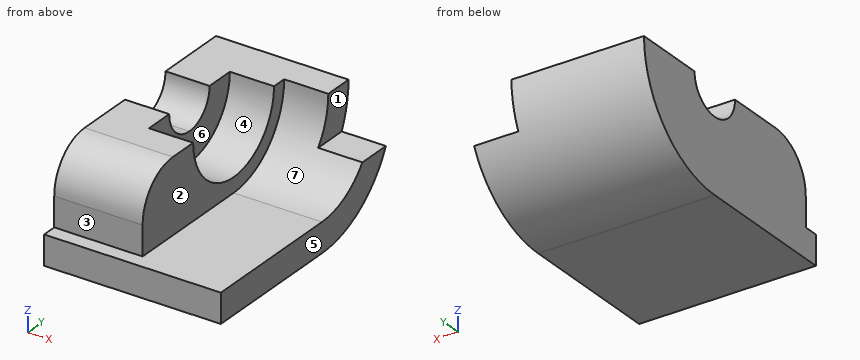
from build123d import *

# Parameters (mm, degrees)
SKETCH1_W           = 2
SKETCH1_H           = 1
BOSS_EXTRUDE1_DEPTH = 12
SKETCH2_W           = 3
SKETCH2_H           = 3
CUT_EXTRUDE1_DEPTH  = 22
CUT_EXTRUDE2_DEPTH  = 6
SKETCH4_R           = 4
CUT_EXTRUDE3_DEPTH  = 3


with BuildPart() as part:
    # Sketch1 → Boss-Extrude1 (new body)
    with BuildSketch(Plane(origin=(0, 0, 0), x_dir=(0, 0, -1), z_dir=(1, 0, 0))):
        with BuildLine():
            Line((1.5, -8), (3.5, -8))
            Line((3.5, -8), (3.5, 1))
            ThreePointArc((3.5, 1), (1.449747468, 5.949747468), (-3.5, 8))
            Line((-3.5, 8), (-3.5, 3))
            ThreePointArc((-3.5, 3), (-2.085786438, 2.414213562), (-1.5, 1))
            ThreePointArc((-1.5, 1), (-2.085786438, -0.414213562), (-3.5, -1))
            Line((-3.5, -1), (-3.5, -5))
            ThreePointArc((-3.5, -5), (-2.621320344, -7.121320344), (-0.5, -8))
            Line((-0.5, -8), (1.5, -8))
        make_face()
        with Locations((2.5, -8.5)):
            Rectangle(SKETCH1_W, SKETCH1_H)
    extrude(amount=BOSS_EXTRUDE1_DEPTH)

    # Sketch2 → Cut-Extrude1 (cut)
    with BuildSketch(Plane.XZ.offset(9)):
        with Locations((10.5, 2)):
            Rectangle(SKETCH2_W, SKETCH2_H)
    extrude(amount=-CUT_EXTRUDE1_DEPTH, mode=Mode.SUBTRACT)

    # Sketch3 → Cut-Extrude2 (cut)
    with BuildSketch(Plane(origin=(12, 0, 0), x_dir=(0, 0, -1), z_dir=(1, 0, 0))):
        with BuildLine():
            Line((1.5, 1), (1.5, -8.778964662))
            ThreePointArc((1.5, -8.778964662), (-3.5, -13.778964662), (-8.5, -8.778964662))
            Line((-8.5, -8.778964662), (-8.5, 1))
            ThreePointArc((-8.5, 1), (-3.5, 6), (1.5, 1))
        make_face()
    extrude(amount=-CUT_EXTRUDE2_DEPTH, mode=Mode.SUBTRACT)

    # Sketch4 → Cut-Extrude3 (cut)
    with BuildSketch(Plane(origin=(6, 0, 0), x_dir=(0, 0, -1), z_dir=(1, 0, 0))):
        with Locations((-3.5, 1)):
            Circle(SKETCH4_R)
    extrude(amount=-CUT_EXTRUDE3_DEPTH, mode=Mode.SUBTRACT)


solid = part.part
Design review of the part built by this model. Coordinates are the model's own, in mm. Face numbers are marked on the shaded views. A direction names the side the tool comes from. Round coordinates to 2 decimals unless told otherwise and drop trailing zeros. Write each loop counter-clockwise with the first axis right and the second up, starting at its lowest first coordinate (ties: lowest second). Pieces come first, ordered by that corner, then holes.
Item 1: Wall thickness on L1, parallel to Z at x = 10.5, y = -3; L2, parallel to Y at x = 4.25, z = 2.75; L3, parallel to X at y = -4.75, z = 0.25: over which ranges is each line inside the solid? List them lowest first.
Item 2: Consider section A-A on z = 3. Give the boundary of the cut face in (x, y), and give its area (3 significant figures).
Item 3: For pin 1 Ø1 at (x, z) = (9, 2) entering from -Y; pin 2 Ø3 at (y, z) = (3, 1.5) entering from +X; pin 3 Ø1.6 at (x, z) = (2, -0.5) entering from -Y, all flat-tipped, find the tip position at first contact; note any pin that passes through.
Item 4: Consider section D-D on x = 6.5. Give the boundary of the cut face in (y, z).
Item 5: Draft analysis for pull direction Y (two halves, no side actions). For the marked faces 5, 6 and 7, state which applies: released by +Y, released by -Y, zero draft, split by the parting line, or undercut.
Item 6: For the marked faces 1, 2, 3 and 4, list the 3-axis set-ups (+Z, -Z, +X, -X, +Y, -Y) from which the entire face can be reached by the end or side of a thin tool; tool diameter is ignored.
Item 7: Consider section C-C on y = -4. Give the boundary of the cut face in (x, z), and give its area (3 significant figures).
Item 8: Consider section B-B on x = 4.5. Give the boundary of the cut face in (y, z).
Check values:
1. L1: z = -3.5 to -1.5
1. L2: y = -6.98 to -2.93, 4.93 to 7.96
1. L3: x = 0 to 6
2. outline: (0, -6.66) - (6, -6.66) - (6, -2.97) - (3, -2.97) - (3, -0.94) - (0, -0.94) - close; (0, 2.94) - (3, 2.94) - (3, 4.97) - (6, 4.97) - (6, 5.97) - (9, 5.97) - (9, 7.98) - (0, 7.98) - close
2. area: 58.4 mm2
3. pin 1: stops at y = 5.58
3. pin 2: stops at x = 6
3. pin 3: stops at y = -8
4. outline: (-9, -3.5) - (1, -3.5) arc R7 ccw to (8, 3.5) - (6, 3.5) arc R5 cw to (1, -1.5) - (-9, -1.5) - close
5. face 5: zero draft
5. face 6: undercut
5. face 7: released by -Y
6. face 1: +Z, +X, +Y, -Y
6. face 2: +Z, +X, -Y
6. face 3: +Z, +X, -X, -Y
6. face 4: +Z, +X
7. outline: (0, -3.5) - (12, -3.5) - (12, -1.5) - (6, -1.5) - (6, 3.5) - (0, 3.5) - close
7. area: 54.0 mm2
8. outline: (-9, -3.5) - (1, -3.5) arc R7 ccw to (8, 3.5) - (5, 3.5) arc R4 cw to (-3, 3.5) - (-5, 3.5) arc R3 ccw to (-8, 0.5) - (-8, -1.5) - (-9, -1.5) - close
